```python
from build123d import *

# Parameters (mm, degrees)
SKETCH1_R       = 5.25
SKETCH1_R_2     = 2.25
MAIN_BODY_DEPTH = 12
CUT_DEPTH       = 15.111165792
CUT_DEPTH_BACK  = 15.111165792
SKETCH3_R       = 0.125


with BuildPart() as part:
    # Sketch1 → Main Body (new body)
    with BuildSketch(Plane(origin=(0, 0, 0), x_dir=(1, 0, 0), z_dir=(0, 1, 0))):
        with Locations(Location((0, 0, 0), (0, 0, 270))):
            Circle(SKETCH1_R)
        with Locations(Location((0, 0, 0), (0, 0, 270))):
            Circle(SKETCH1_R_2, mode=Mode.SUBTRACT)
    extrude(amount=MAIN_BODY_DEPTH)

    # Sketch3 → Cut (cut, two sides: drawn at the far end of the back side and taken through both)
    with BuildSketch(Plane(origin=(0, 12, 0), x_dir=(1, 0, 0), z_dir=(0, 1, 0)).offset(-CUT_DEPTH_BACK)):
        with Locations((0, 5.25)):
            Circle(SKETCH3_R)
        with Locations((0.657999476, 5.208602182)):
            Circle(SKETCH3_R)
        with Locations((1.305621908, 5.085061596)):
            Circle(SKETCH3_R)
        with Locations((1.932653902, 4.881326551)):
            Circle(SKETCH3_R)
        with Locations((2.529206789, 4.60061007)):
            Circle(SKETCH3_R)
        with Locations((3.085872575, 4.24733922)):
            Circle(SKETCH3_R)
        with Locations((3.593872306, 3.827085294)):
            Circle(SKETCH3_R)
        with Locations((4.045194525, 3.346475946)):
            Circle(SKETCH3_R)
        with Locations((4.432721609, 2.813090674)):
            Circle(SKETCH3_R)
        with Locations((4.750342025, 2.235341281)):
            Circle(SKETCH3_R)
        with Locations((4.993046711, 1.62233922)):
            Circle(SKETCH3_R)
        with Locations((5.157008066, 0.983751902)):
            Circle(SKETCH3_R)
        with Locations((5.239640324, 0.329650228)):
            Circle(SKETCH3_R)
        with Locations((5.239640324, -0.329650228)):
            Circle(SKETCH3_R)
        with Locations((5.157008066, -0.983751902)):
            Circle(SKETCH3_R)
        with Locations((4.993046711, -1.62233922)):
            Circle(SKETCH3_R)
        with Locations((4.750342025, -2.235341281)):
            Circle(SKETCH3_R)
        with Locations((4.432721609, -2.813090674)):
            Circle(SKETCH3_R)
        with Locations((4.045194525, -3.346475946)):
            Circle(SKETCH3_R)
        with Locations((3.593872306, -3.827085294)):
            Circle(SKETCH3_R)
        with Locations((3.085872575, -4.24733922)):
            Circle(SKETCH3_R)
        with Locations((2.529206789, -4.60061007)):
            Circle(SKETCH3_R)
        with Locations((1.932653902, -4.881326551)):
            Circle(SKETCH3_R)
        with Locations((1.305621908, -5.085061596)):
            Circle(SKETCH3_R)
        with Locations((0.657999476, -5.208602182)):
            Circle(SKETCH3_R)
        with Locations((0, -5.25)):
            Circle(SKETCH3_R)
        with Locations((-0.657999476, -5.208602182)):
            Circle(SKETCH3_R)
        with Locations((-1.305621908, -5.085061596)):
            Circle(SKETCH3_R)
        with Locations((-1.932653902, -4.881326551)):
            Circle(SKETCH3_R)
        with Locations((-2.529206789, -4.60061007)):
            Circle(SKETCH3_R)
        with Locations((-3.085872575, -4.24733922)):
            Circle(SKETCH3_R)
        with Locations((-3.593872306, -3.827085294)):
            Circle(SKETCH3_R)
        with Locations((-4.045194525, -3.346475946)):
            Circle(SKETCH3_R)
        with Locations((-4.432721609, -2.813090674)):
            Circle(SKETCH3_R)
        with Locations((-4.750342025, -2.235341281)):
            Circle(SKETCH3_R)
        with Locations((-4.993046711, -1.62233922)):
            Circle(SKETCH3_R)
        with Locations((-5.157008066, -0.983751902)):
            Circle(SKETCH3_R)
        with Locations((-5.239640324, -0.329650228)):
            Circle(SKETCH3_R)
        with Locations((-5.239640324, 0.329650228)):
            Circle(SKETCH3_R)
        with Locations((-5.157008066, 0.983751902)):
            Circle(SKETCH3_R)
        with Locations((-4.993046711, 1.62233922)):
            Circle(SKETCH3_R)
        with Locations((-4.750342025, 2.235341281)):
            Circle(SKETCH3_R)
        with Locations((-4.432721609, 2.813090674)):
            Circle(SKETCH3_R)
        with Locations((-4.045194525, 3.346475946)):
            Circle(SKETCH3_R)
        with Locations((-3.593872306, 3.827085294)):
            Circle(SKETCH3_R)
        with Locations((-3.085872575, 4.24733922)):
            Circle(SKETCH3_R)
        with Locations((-2.529206789, 4.60061007)):
            Circle(SKETCH3_R)
        with Locations((-1.932653902, 4.881326551)):
            Circle(SKETCH3_R)
        with Locations((-1.305621908, 5.085061596)):
            Circle(SKETCH3_R)
        with Locations((-0.657999476, 5.208602182)):
            Circle(SKETCH3_R)
    extrude(amount=CUT_DEPTH + CUT_DEPTH_BACK, mode=Mode.SUBTRACT)


solid = part.part
```
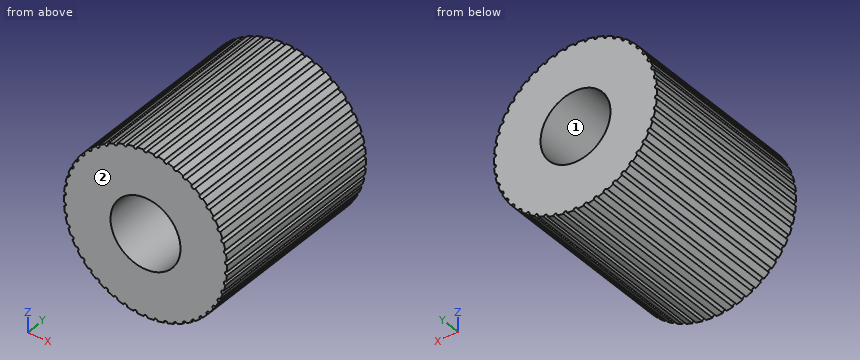
Part model, mm, in its own coordinate system. Face numbers are marked on the shaded views. Round coordinates to 2 decimals unless told otherwise and drop trailing zeros. Write each loop counter-clockwise with the first axis right and the second up, starting at its lowest first coordinate (ties: lowest second). Pieces come first, ordered by that corner, then holes. Notation, with made-up numbers: (49, 32) -> (100, 32) arc R35 ccw to (100, 65) -> close; hole circle Ø7 at (-25, -13). An arc over 180 degrees is marked (long way). Return JSON: item names as keys, results as strings. Group by question number.
Q1. Pin check, flat tips, straight feed: pin 1 (5 mm diameter, centred on x = 2.5, y = 6.5, fed in from +Z); pin 2 (1.5 mm diameter, centred on x = -2.5, y = 6, fed in from -Z); pin 3 (3 mm diameter, centred on x = 3, y = 2, fed in from +Z). Stop position of each tip, or through.
Q2. Saw through at B-B on x = 1. Write the cut outline in (y, z), plus the area to 3 significant figures.
Q3. Saw through at A-A on z = 0. Write the cut outline in (x, y).
Q4. Probe L1, parallel to X at y = 2.5, z = 0; L2, parallel to Z at x = 0.5, y = 7.5; L3, parallel to Z at x = -2.75, y = 6.25. List the from-to ranges inside material, lowest first. Write a range as [from, to].
Q5. Mould opens along X. For the marked faces 1 and 2 say: pulls with the +X half, pulls with the -X half, needs draft (parallel to the pull), parting line crosses it, or undercut.
Answer:
{
 "1": {"pin 1": "z = 5.25", "pin 2": "z = -4.95", "pin 3": "z = 5.03"},
 "2": {"outline": "(0, -5.15) -> (12, -5.15) -> (12, -2.02) -> (0, -2.02) -> close; (0, 2.02) -> (12, 2.02) -> (12, 5.15) -> (0, 5.15) -> close", "area": "75.3 mm2"},
 "3": {"outline": "(-5.25, 0) -> (-2.25, 0) -> (-2.25, 12) -> (-5.25, 12) -> close; (2.25, 0) -> (5.25, 0) -> (5.25, 12) -> (2.25, 12) -> close"},
 "4": {"L1": "[-5.25, -2.25], [2.25, 5.25]", "L2": "[-5.23, -2.19], [2.19, 5.23]", "L3": "[-4.47, 4.47]"},
 "5": {"face 1": "undercut", "face 2": "needs draft"}
}
